Could you check a few things on this model? Use its own coordinates, in mm. Face numbers are marked on the shaded views. A direction names the side the tool comes from. Round coordinates to 2 decimals unless told otherwise and drop trailing zeros. Loops run counter-clockwise (first coordinate to the right, second up) from the corner with the lowest first, then second, coordinate; pieces in that order, holes last. Notation, with made-up numbers: (-0.75, 50.5) -> (55.25, 50.5) arc R10 cw to (55.25, 67.5) -> close; hole circle Ø6 at (-10, 39). An arc over 180 degrees is marked (long way). Use CSV: the item, a comma, the result in double quotes. Start each with the question number.
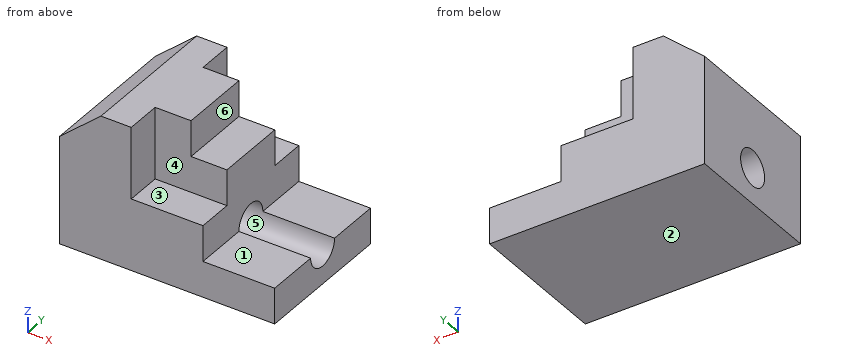
```python
from build123d import *

# Parameters (mm, degrees)
F1_DEPTH = 50.8
F3_DEPTH = 12.7
F5_START = 38.1
F5_DEPTH = 12.701
F6_R     = 6.35
F7_DEPTH = 76.201


with BuildPart() as f1:
    # F0 (on Front) → F1 (new body)
    with BuildSketch(Plane.XZ):
        Polygon((0, 38.1), (0, 0), (76.2, 0), (76.2, 12.7), (50.8, 12.7), (50.8, 38.1), (38.1, 38.1), (38.1, 50.8), (14.6706935452, 50.8), align=None)
    extrude(amount=F1_DEPTH)

    # F2 (on Front) → F3 (cut)
    with BuildSketch(Plane.XZ):
        Polygon((38.1, 50.8), (25.4, 50.8), (25.4, 25.4), (50.8, 25.4), (50.8, 38.1), (38.1, 38.1), align=None)
    extrude(amount=F3_DEPTH, mode=Mode.SUBTRACT)

    # F4 (on Front) → F5 (cut)
    with BuildSketch(Plane.XZ.offset(F5_START)):
        Polygon((38.1, 50.8), (25.4, 50.8), (25.4, 25.4), (50.8, 25.4), (50.8, 38.1), (38.1, 38.1), align=None)
    extrude(amount=F5_DEPTH, mode=Mode.SUBTRACT)

    # F6 (on Right) → F7 (cut, through all)
    with BuildSketch(Plane.YZ):
        with Locations((-25.4, 12.7)):
            Circle(F6_R)
    extrude(amount=F7_DEPTH, mode=Mode.SUBTRACT)


solid = f1.part
```
1. Suppose I cut it at C-C (x = 22.5). List the corners of the cut face in (y, z) for me.
2. Suppose I cut it at A-A (y = -25.4). List the corners of the cut face in (x, z) for me.
3. Will these pins go through, and if not, where does the flat tip stop? pin 1 (15 mm diameter, centred on x = 65.5, y = -5, fed in from +Z); pin 2 (4 mm diameter, centred on x = 41, y = -5, fed in from +Z); pin 3 (7.5 mm diameter, centred on y = -21, z = 21, fed in from +X).
4. Suppose I cut it at B-B (y = -39). List the corners of the cut face in (x, z) for me.
5. We'd pull the mould along Y, two halves only. Please class the marked faces 4, 5 and 6: pulls with the +Y half, pulls with the -Y half, needs draft (parallel to the pull), parting line crosses it, or undercut.
6. Suppose I cut it at D-D (z = 22.5). List the corners of the cut face in (x, y) for me, then the cut area to 3 significant figures.
7. For the marked faces 1, 2 and 3, which set-ups out of +Z, -Z, +X, -X, +Y, -Y let a thin tool reach every point of the face, with its end or its side?
8. If I drill on L1, parallel to Y at x = 21.5, z = 12.7; L2, parallel to Z at x = 36.5, y = -25.4; L3, parallel to Z at x = 49, y = -2.5, over which ranges is the centre line in solid material (lowest first)?
Geometry check:
1,outline,"(-50.8, 0) -> (0, 0) -> (0, 50.8) -> (-50.8, 50.8) -> close; hole circle Ø12.7 at (-25.4, 12.7)"
2,outline,"(0, 0) -> (76.2, 0) -> (76.2, 6.35) -> (0, 6.35) -> close; (0, 19.05) -> (50.8, 19.05) -> (50.8, 38.1) -> (38.1, 38.1) -> (38.1, 50.8) -> (14.67, 50.8) -> (0, 38.1) -> close"
3,pin 1,"stops at z = 12.7"
3,pin 2,"stops at z = 25.4"
3,pin 3,"stops at x = 50.8"
4,outline,"(0, 0) -> (76.2, 0) -> (76.2, 12.7) -> (50.8, 12.7) -> (50.8, 25.4) -> (25.4, 25.4) -> (25.4, 50.8) -> (14.67, 50.8) -> (0, 38.1) -> close"
5,face 4,"pulls with the -Y half"
5,face 5,"undercut"
5,face 6,"needs draft"
6,outline,"(0, -50.8) -> (50.8, -50.8) -> (50.8, 0) -> (0, 0) -> close"
6,area,"2,580 mm²"
7,face 1,"+Z, +X, +Y, -Y"
7,face 2,"-Z, +X, -X, +Y, -Y"
7,face 3,"+Z, +X, -Y"
8,L1,"y = -50.8 to -31.75, -19.05 to 0"
8,L2,"z = 0 to 6.35, 19.05 to 50.8"
8,L3,"z = 0 to 25.4"
